```python
from build123d import *

# Parameters (mm, degrees)
F0_R     = 10
F1_DEPTH = 11
F2_R     = 5
F3_DEPTH = 8
F5_D     = 6
F5_DEPTH = 12
F5_TIP   = 1.8025818571
F6_SIZE  = 2


with BuildPart() as f1:
    # F0 (on Top) → F1 (new body)
    with BuildSketch(Plane.XY):
        Circle(F0_R)
    extrude(amount=F1_DEPTH)

    # F2 (on face) → F3 (join)
    with BuildSketch(Plane.XY.offset(11)):
        Circle(F2_R)
    extrude(amount=F3_DEPTH)

    # F5
    with Locations(Plane.XY.offset(19)):
        with Locations((0, 0)):
            Hole(F5_D / 2, depth=F5_DEPTH)
            with Locations((0, 0, -(F5_DEPTH + F5_TIP / 2))):  # 118° drill point
                Cone(0, F5_D / 2, F5_TIP, mode=Mode.SUBTRACT)

    # F6
    f6_edges = [f1.edges().sort_by_distance(p)[0] for p in [
        (-10, 0, 0),
    ]]
    chamfer(f6_edges, length=F6_SIZE)


solid = f1.part
```
Geometry check sheet. Reference: the model listing, model coordinates, mm. A direction names the side the tool comes from. Round coordinates to 2 decimals unless told otherwise and drop trailing zeros. Loops run counter-clockwise (first coordinate to the right, second up) from the corner with the lowest first, then second, coordinate; pieces in that order, holes last. Notation, with made-up numbers: (-37, 67.5) - (-31, 67.5) arc R37 ccw to (-31, 104.5) - close; hole circle Ø3 at (19, -38.5). An arc over 180 degrees is marked (long way). Write item = value, one per line. Start each with the question number.
1. Mould release check, pull along X, two halves, no side actions. Record for faces 3 (the face through (0, 0, 0)), 4 (the face through (-2.17, -9.76, 6.44)), 5 (the face through (0.24, -0.46, 5.51)): released by +X, released by -X, zero draft, split by the parting line, or undercut.
2. Section check A-A on z = 7.5. Enter the section's corners in (x, y), then the cut area to 3 significant figures.
3. Section check B-B on z = 16.75. Enter the section's corners in (x, y), then the cut area to 3 significant figures.
4. Set-up check for faces 1 (the face through (-1.08, -4.88, 14.94)), 2 (the face through (-0.1, -3.3, 19)): record each of +Z, -Z, +X, -X, +Y, -Y from which the full face is reachable in a straight line by a thin tool's end or side.
5. Thickness scan on line 1 (Y direction, x = 0, z = 14.5); line 2 (Z direction, x = -4.25, y = 4.5); line 3 (Y direction, x = 0, z = 10.5). Record the ranges inside material, lowest first.
6. Depth check by flat-ended pin: pin 1 (3 mm diameter, centred on x = -8, z = 2.5, fed in from -Y); pin 2 (4 mm diameter, centred on x = 4.5, z = 13.5, fed in from -Y); pin 3 (1 mm diameter, centred on y = -5.5, z = 11, fed in from -X). Enter the tip coordinate at first touch or a pass-through.
Working result:
q1.face_3 = zero draft
q1.face_4 = split by the parting line
q1.face_5 = undercut
q2.outline = circle Ø20 at (0, 0); hole circle Ø6 at (0, 0)
q2.area = 286 mm^2
q3.outline = circle Ø10 at (0, 0); hole circle Ø6 at (0, 0)
q3.area = 50.3 mm^2
q4.face_1 = +Z
q4.face_2 = +Z, +X, -X, +Y, -Y
q5.line_1 = -5 to -3, 3 to 5
q5.line_2 = 0 to 11
q5.line_3 = -10 to -3, 3 to 10
q6.pin_1 = -7.6
q6.pin_2 = -4.33
q6.pin_3 = -8.66
